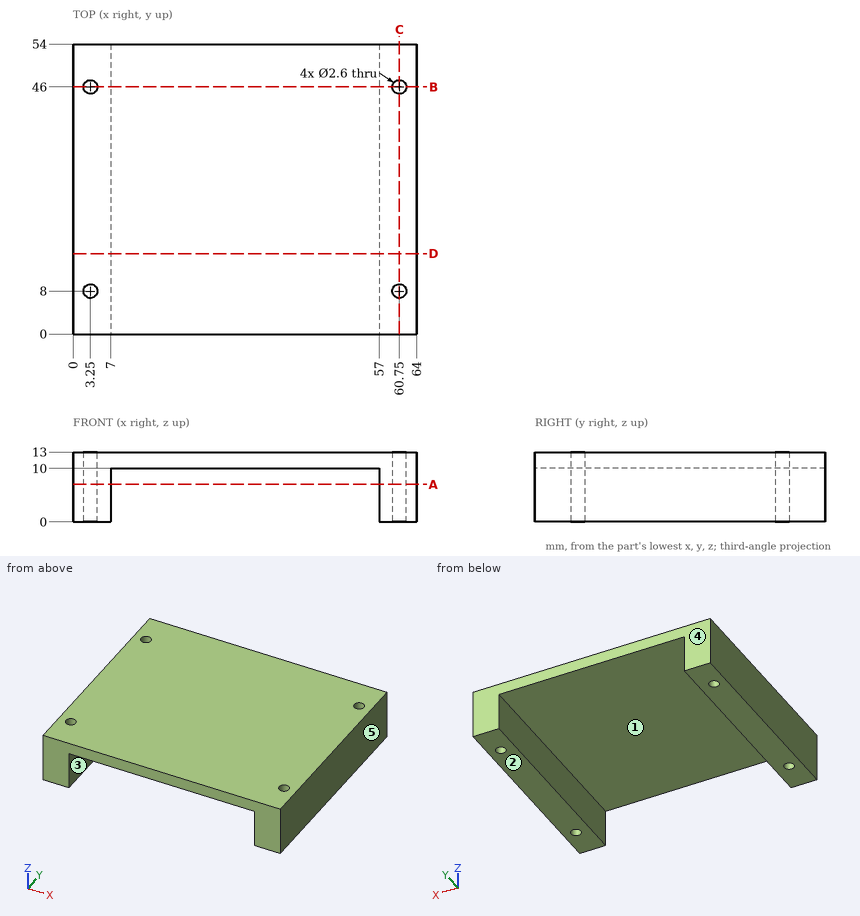
Design review of the part shown in the three views and the two pictorial views. Dimensions are in mm from the part's minimum x, y and z. A direction names the side the tool comes from. Give positions to 0.01 mm unless a question says otherwise; leave off trailing zeros. Loops run counter-clockwise (first coordinate to the right, second up) from the corner with the lowest first, then second, coordinate; pieces in that order, holes last. Notation, with made-up numbers: (67, 1.25) -> (93, 1.25) arc R20 ccw to (93, 28.25) -> close; hole circle Ø4 at (17, 64.25). An arc over 180 degrees is marked (long way). Write each question's results on one line, items separated by ' | '.
Q1. Machinability: for the marked faces 1 and 2, which of the approach directions +Z, -Z, +X, -X, +Y, -Y give a long, thin tool a straight path to every point of the face, cutting with its end or side? Answer none if there is none.
Reply:
face 1: -Z, +Y, -Y | face 2: -Z, +X, -X, +Y, -Y
Q2. The part is to be moulded in two halves that separate along X. For the marked faces 3, 4 and 5, say which applies: +X half, -X half, draft (parallel to the pull), parting line (faces both ways), or undercut.
Reply:
face 3: undercut | face 4: draft | face 5: +X half
Q3. For pin 1 Ø1.6 at (x, y) = (60.75, 8) entering from +Z; pin 2 Ø15 at (x, y) = (37, 29.5) entering from -Z, all flat-tipped, find the tip position at first contact; note any pin that passes through.
Reply:
pin 1: passes through | pin 2: stops at z = 10
Q4. Take a section at D-D, the plane y = 15. Write out the cut boundary in (x, z), plus the area to 3 significant figures.
Reply:
outline: (0, 0) -> (7, 0) -> (7, 10) -> (57, 10) -> (57, 0) -> (64, 0) -> (64, 13) -> (0, 13) -> close | area: 332 mm²
Q5. Wall thickness on L1, parallel to X at y = 46, z = 9.5; L2, parallel to Y at x = 3.25, z = 6.25; L3, parallel to X at y = 34.5, z = 9.25: over which ranges is each line inside the solid? List them lowest first.
Reply:
L1: x = 0 to 1.95, 4.55 to 7, 57 to 59.45, 62.05 to 64 | L2: y = 0 to 6.7, 9.3 to 44.7, 47.3 to 54 | L3: x = 0 to 7, 57 to 64
Q6. Take a section at B-B, the plane y = 46. Write out the cut boundary in (x, z), plus the area to 3 significant figures.
Reply:
outline: (0, 0) -> (1.95, 0) -> (1.95, 13) -> (0, 13) -> close; (4.55, 0) -> (7, 0) -> (7, 10) -> (57, 10) -> (57, 0) -> (59.45, 0) -> (59.45, 13) -> (4.55, 13) -> close; (62.05, 0) -> (64, 0) -> (64, 13) -> (62.05, 13) -> close | area: 264 mm²
Q7. Take a section at C-C, the plane x = 60.75. Write out the cut boundary in (y, z), plus the area to 3 significant figures.
Reply:
outline: (0, 0) -> (6.7, 0) -> (6.7, 13) -> (0, 13) -> close; (9.3, 0) -> (44.7, 0) -> (44.7, 13) -> (9.3, 13) -> close; (47.3, 0) -> (54, 0) -> (54, 13) -> (47.3, 13) -> close | area: 634 mm²
Q8. Take a section at A-A, the plane z = 7. Write out the cut boundary in (x, y), plus the area to 3 significant figures.
Reply:
outline: (0, 0) -> (7, 0) -> (7, 54) -> (0, 54) -> close; (57, 0) -> (64, 0) -> (64, 54) -> (57, 54) -> close; hole circle Ø2.6 at (3.25, 8); hole circle Ø2.6 at (3.25, 46); hole circle Ø2.6 at (60.75, 8); hole circle Ø2.6 at (60.75, 46) | area: 735 mm²
